Verification items for the finished model (mm, model axes). Round coordinates to 2 decimals unless told otherwise and drop trailing zeros. Write each loop counter-clockwise with the first axis right and the second up, starting at its lowest first coordinate (ties: lowest second). Pieces come first, ordered by that corner, then holes. Notation, with made-up numbers: (12, -6) - (66, -6) arc R21 ccw to (66, 20) - close; hole circle Ø6 at (-8, -20.75). An arc over 180 degrees is marked (long way). Answer as a JSON object with one key per item and string values. Group by question number.
1) Mould release check, pull along Y, two halves, no side actions. Record for faces 1 (the cylindrical face through (0.182, -3.68, 11.684)), 2 (the cylindrical face through (0.182, -6.083, -6.633)), 3 (the flat face through (13.5, 0, -10)): +Y half, -Y half, draft (parallel to the pull), parting line (faces both ways), or undercut.
2) Section check A-A (z = 0). Enter the section's corners in (x, y), then the cut area to 4 significant figures.
3) Thickness scan on line 1 (Y direction, x = 3.5, z = 0); line 2 (Z direction, x = 5.75, y = -7); line 3 (Z direction, x = 4, y = 7.5). Record the ranges inside material, lowest first.
4) Section check C-C (x = 1). Enter the section's corners in (y, z).
5) Go/stop test with flat-tipped pins: pin 1 Ø8 at (y, z) = (2, -0.5) entering from +X; pin 2 Ø1.5 at (y, z) = (4.5, 7) entering from +X; pin 3 Ø1.5 at (x, y) = (-0.5, -7.5) entering from -Z; pin 4 Ø1 at (x, y) = (-4, -6) entering from -Z. Record where each tip stops, or that it passes through.
```python
from build123d import *

# Parameters (mm, degrees)
ESQUISSE1_W     = 27
ESQUISSE1_H     = 3.25
CHANFREIN1_SIZE = 0.5


with BuildPart() as part:
    # Esquisse1 → Base-Révol.-Mince (revolve)
    with BuildSketch(Plane.XY, mode=Mode.PRIVATE) as base_r_vol_mince_sk:
        with Locations((0, 10.625)):
            Rectangle(ESQUISSE1_W, ESQUISSE1_H)
    revolve(base_r_vol_mince_sk.sketch.rotate(Axis((0, 0, 0), (1, 0, 0)), 90), axis=Axis((0, 0, 0), (1, 0, 0)))

    # Chanfrein1
    chanfrein1_edges = [part.edges().sort_by_distance(p)[0] for p in [
        (-13.5, 0, -12.25),
        (13.5, 0, -12.25),
        (13.5, 0, -9),
        (-13.5, 0, -9),
    ]]
    chamfer(chanfrein1_edges, length=CHANFREIN1_SIZE)


solid = part.part
```
Returned:
{
 "1": {"face 1": "parting line", "face 2": "undercut", "face 3": "draft"},
 "2": {"outline": "(-13.5, -11.75) - (-13, -12.25) - (13, -12.25) - (13.5, -11.75) - (13.5, -9.5) - (13, -9) - (-13, -9) - (-13.5, -9.5) - close; (-13.5, 9.5) - (-13, 9) - (13, 9) - (13.5, 9.5) - (13.5, 11.75) - (13, 12.25) - (-13, 12.25) - (-13.5, 11.75) - close", "area": "174.5 mm2"},
 "3": {"line 1": "-12.25 to -9, 9 to 12.25", "line 2": "-10.05 to -5.66, 5.66 to 10.05", "line 3": "-9.69 to -4.97, 4.97 to 9.69"},
 "4": {"outline": "circle Ø24.5 at (0, 0); hole circle Ø18 at (0, 0)"},
 "5": {"pin 1": "through", "pin 2": "x = 13.07", "pin 3": "z = -10.22", "pin 4": "z = -10.95"}
}
